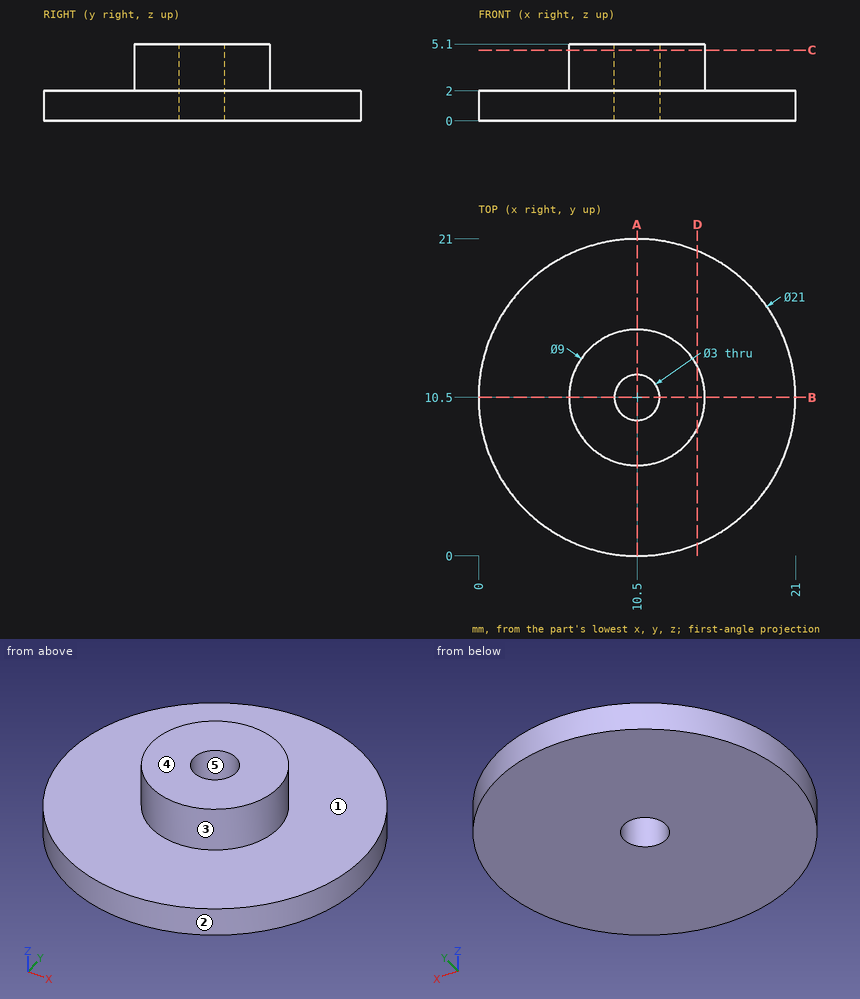
Check sheet for the drawn part. Datum: minimum x, y, z corner. Units: mm. A direction names the side the tool comes from. Round coordinates to 2 decimals unless told otherwise and drop trailing zeros. Loops run counter-clockwise (first coordinate to the right, second up) from the corner with the lowest first, then second, coordinate; pieces in that order, holes last. Notation, with made-up numbers: (17, 41.5) - (59, 41.5) arc R24 ccw to (59, 57.5) - close; hole circle Ø10 at (41, 79.25). An arc over 180 degrees is marked (long way). Use one line per item in the form item = value.
1. Scan lines: probe 1 along Y at (x, z) = (10.5, 1.05); probe 2 along Z at (x, y) = (4, 16); probe 3 along Y at (x, z) = (10.5, 3.8). Record each from-to range of solid material in increasing order.
A:
probe_1 = 0 to 9, 12 to 21
probe_2 = 0 to 2
probe_3 = 6 to 9, 12 to 15
2. Section check A-A on x = 10.5. Record the cut outline in (y, z).
A:
outline = (0, 0) - (9, 0) - (9, 5.1) - (6, 5.1) - (6, 2) - (0, 2) - close; (12, 0) - (21, 0) - (21, 2) - (15, 2) - (15, 5.1) - (12, 5.1) - close
3. Gauge pin test, flat ends, axial feed: pin 1 Ø1.5 at (x, z) = (12.5, 2.5) entering from -Y; pin 2 Ø1.5 at (x, y) = (16, 10.5) entering from +Z. Record the tip position at first contact, or that the pin passes through.
A:
pin_1 = 0.1
pin_2 = 2
4. Section check C-C on z = 4.7. Record the cut outline in (x, y).
A:
outline = circle Ø9 at (10.5, 10.5); hole circle Ø3 at (10.5, 10.5)
5. Section check D-D on x = 14.5. Record the cut outline in (y, z).
A:
outline = (0.79, 0) - (20.21, 0) - (20.21, 2) - (12.56, 2) - (12.56, 5.1) - (8.44, 5.1) - (8.44, 2) - (0.79, 2) - close
6. Access from +Z, -Z, +X, -X, +Y, -Y to the whole of each face (thin tool, end or side, straight path). Record for the marked faces 1 and 2.
A:
face_1 = +Z
face_2 = +Z, -Z
7. Draft check along Y on the marked faces 3, 4 and 5. Enter one of: pulls with the +Y half, pulls with the -Y half, needs draft (parallel to the pull), parting line crosses it, or undercut.
A:
face_3 = parting line crosses it
face_4 = needs draft
face_5 = undercut
